The listing builds one solid part. Answer for the finished solid, in the listing's coordinates (mm). A direction names the side the tool comes from. Round coordinates to 2 decimals unless told otherwise and drop trailing zeros. Loops run counter-clockwise (first coordinate to the right, second up) from the corner with the lowest first, then second, coordinate; pieces in that order, holes last. Notation, with made-up numbers: (10.5, 38.5) -> (49.5, 38.5) arc R11 cw to (49.5, 43.5) -> close; hole circle Ø10 at (46, 20.25). An arc over 180 degrees is marked (long way). Write each question's results on one line, items separated by ' | '. Start each with the question number.
(1) Determine the mould class of faces 5 (the face through (-217.395, 142.762, 75.151)), 6 (the face through (-260, 125, -20)), 7 (the face through (-217.4, 145.64, 81.16)) for opening direction Y: released by +Y, released by -Y, zero draft, split by the parting line, or undercut.
(2) Straight lines are drawn through the part: probe 1 along Y at (x, z) = (-214.5, 75); probe 2 along Z at (x, y) = (40.5, 15.5); probe 3 along X at (y, z) = (56, 48). For each, find the intervals that lie inside material, in ascending order.
(3) The part is cut by section D-D (z = -31). Determine the outline of the cut face in (x, y).
(4) The part is cut by section A-A (y = 121.5). Determine the outline of the cut face in (x, z), plus the area to 3 significant figures.
(5) For faces 1 (the face through (205, 120, 80)), 2 (the face through (-205, 135, 75)), 3 (the face through (-205, 105, 75)), 4 (the face through (-210, 143, 77)), determine the directions among +Z, -Z, +X, -X, +Y, -Y from which every point of the face is accessible in a straight line to the end or side of a thin tool.
(6) The part is cut by section C-C (x = -84). Determine the outline of the cut face in (y, z).
(7) Flat-ended cylindrical pins translate along their axes: pin 1 (3 mm diameter, centred on y = 114.5, z = 76, fed in from -X); pin 2 (1 mm diameter, centred on x = 46.5, z = -41, fed in from +Y); pin 3 (24 mm diameter, centred on x = -195.5, y = 113.5, fed in from +Z). Find the tip coordinate at first contact, or state that the pin passes through.
(8) The part is cut by section B-B (y = 65.5). Determine the outline of the cut face in (x, z).
```python
from build123d import *

# Parameters (mm, degrees)
SKETCH_1_W          = 540
SKETCH_1_H          = 140
EXTRUDE_1_DEPTH     = 140
SKETCH_2_W          = 500
SKETCH_2_H          = 100
CUT_EXTRUDE_1_DEPTH = 150
SKETCH_4_W          = 40
SKETCH_4_H          = 30
EXTRUDE_2_DEPTH     = 30
SKETCH_5_W          = 40
SKETCH_5_H          = 30
EXTRUDE_3_DEPTH     = 30
SKETCH_7_R          = 10
SKETCH_7_R_2        = 5
EXTRUDE_1_2_DEPTH   = 15
EXTRUDE_START       = -15
SKETCH_9_R          = 10
SKETCH_9_R_2        = 5
EXTRUDE_2_2_DEPTH   = 15
SKETCH_11_W         = 40
SKETCH_11_H         = 30
CUT_EXTRUDE_3_DEPTH = 567.267937246
SKETCH_13_W         = 540
SKETCH_13_H         = 140
EXTRUDE_6_DEPTH     = 30


with BuildPart() as part:
    # 草圖1 → Extrude 1 (new body)
    with BuildSketch(Plane(origin=(0, 0, 0), x_dir=(1, 0, 0), z_dir=(0, 1, 0))):
        Rectangle(SKETCH_1_W, SKETCH_1_H)
    extrude(amount=EXTRUDE_1_DEPTH)

    # 草圖2 → 除料-伸長1 (cut)
    with BuildSketch(Plane(origin=(0, 140, 0), x_dir=(1, 0, 0), z_dir=(0, 1, 0))):
        Rectangle(SKETCH_2_W, SKETCH_2_H)
    extrude(amount=-CUT_EXTRUDE_1_DEPTH, mode=Mode.SUBTRACT)

    # 草圖4 → Extrude 2 (add)
    with BuildSketch(Plane.XY.offset(80)):
        with Locations((-205, 120)):
            Rectangle(SKETCH_4_W, SKETCH_4_H)
    extrude(amount=-EXTRUDE_2_DEPTH)

    # 草圖5 → 填料-伸長3 (add)
    with BuildSketch(Plane.XY.offset(80)):
        with Locations((205, 120)):
            Rectangle(SKETCH_5_W, SKETCH_5_H)
    extrude(amount=-EXTRUDE_3_DEPTH)

    # 草圖7 → Extrude 1 2 (add)
    with BuildSketch(Plane(origin=(225, 0, 0), x_dir=(0, 0, -1), z_dir=(1, 0, 0))):
        with Locations((-75, 137.764599119)):
            Circle(SKETCH_7_R)
        with Locations((-75, 137.764599119)):
            Circle(SKETCH_7_R_2, mode=Mode.SUBTRACT)
    extrude(amount=-EXTRUDE_1_2_DEPTH)

    # 草圖9 → Extrude 2 2 (add)
    with BuildSketch(Plane.ZY.offset(225).offset(EXTRUDE_START)):
        with Locations((75, 137.764599119)):
            Circle(SKETCH_9_R)
        with Locations((75, 137.764599119)):
            Circle(SKETCH_9_R_2, mode=Mode.SUBTRACT)
    extrude(amount=EXTRUDE_2_2_DEPTH)

    # 草圖11 → 除料-伸長3 (cut, through all)
    with BuildSketch(Plane.ZY.offset(270)):
        with Locations((0, 125)):
            Rectangle(SKETCH_11_W, SKETCH_11_H)
    extrude(amount=-CUT_EXTRUDE_3_DEPTH, mode=Mode.SUBTRACT)

    # 草圖13 → 填料-伸長6 (add)
    with BuildSketch(Plane.XZ):
        Rectangle(SKETCH_13_W, SKETCH_13_H)
    extrude(amount=EXTRUDE_6_DEPTH)


solid = part.part
```
Checked values:
1) face 5: undercut | face 6: zero draft | face 7: split by the parting line
2) probe 1: y = 105 to 135, 142.76 to 147.76 | probe 2: z = -70 to -50, 50 to 70 | probe 3: x = -270 to -250, 250 to 270
3) outline: (-270, -30) -> (270, -30) -> (270, 140) -> (250, 140) -> (250, 0) -> (-250, 0) -> (-250, 140) -> (-270, 140) -> close
4) outline: (-270, -70) -> (270, -70) -> (270, -20) -> (250, -20) -> (250, -50) -> (-250, -50) -> (-250, -20) -> (-270, -20) -> close; (-270, 20) -> (-250, 20) -> (-250, 50) -> (250, 50) -> (250, 20) -> (270, 20) -> (270, 70) -> (225, 70) -> (225, 80) -> (185, 80) -> (185, 70) -> (-185, 70) -> (-185, 80) -> (-225, 80) -> (-225, 70) -> (-270, 70) -> close | area: 24,800 mm2
5) face 1: +Z, -Y | face 2: none | face 3: +Z, +X, -X, -Y | face 4: +Z, +Y
6) outline: (-30, -70) -> (140, -70) -> (140, -50) -> (0, -50) -> (0, 50) -> (140, 50) -> (140, 70) -> (-30, 70) -> close
7) pin 1: stops at x = -225 | pin 2: stops at y = 0 | pin 3: stops at z = 80
8) outline: (-270, -70) -> (270, -70) -> (270, 70) -> (-270, 70) -> close; hole (-250, -50) -> (250, -50) -> (250, 50) -> (-250, 50) -> close
